```python
from build123d import *

# Parameters (mm, degrees)
ESQUISSE1_R             = 4
EXTRUSION1_DEPTH        = 5
ENL_V_MAT_EXTRU_1_DEPTH = 2
CONG_1_R                = 2.5


with BuildPart() as part:
    # Esquisse1 → Extrusion1 (new body)
    with BuildSketch(Plane.XY):
        with BuildLine():
            Line((-8, 0), (8, 0))
            ThreePointArc((8, 0), (10.121320344, 0.878679656), (11, 3))
            Line((11, 3), (11, 37))
            ThreePointArc((11, 37), (8, 40), (11, 43))
            Line((11, 43), (11, 78))
            ThreePointArc((11, 78), (10.121320344, 80.121320344), (8, 81))
            Line((8, 81), (-8, 81))
            ThreePointArc((-8, 81), (-10.121320344, 80.121320344), (-11, 78))
            Line((-11, 78), (-11, 3))
            ThreePointArc((-11, 3), (-10.121320344, 0.878679656), (-8, 0))
        make_face()
        with Locations((0, 9)):
            Circle(ESQUISSE1_R, mode=Mode.SUBTRACT)
        with Locations((0, 30)):
            Circle(ESQUISSE1_R, mode=Mode.SUBTRACT)
        with Locations((0, 50)):
            Circle(ESQUISSE1_R, mode=Mode.SUBTRACT)
        with Locations((0, 70)):
            Circle(ESQUISSE1_R, mode=Mode.SUBTRACT)
    extrude(amount=EXTRUSION1_DEPTH)

    # Esquisse2 → Enlèv. mat.-Extru.1 (cut)
    with BuildSketch(Plane.XY.offset(5)):
        with BuildLine():
            Line((4, 75.744562647), (4, 64.255437353))
            ThreePointArc((4, 64.255437353), (0, 63), (-4, 64.255437353))
            Line((-4, 64.255437353), (-4, 75.744562647))
            ThreePointArc((-4, 75.744562647), (0, 77), (4, 75.744562647))
        make_face()
    extrude(amount=-ENL_V_MAT_EXTRU_1_DEPTH, mode=Mode.SUBTRACT)

    # Congé1
    # the kernel refuses this fillet: 2.5 mm, written as the material it takes off along each edge
    with BuildSketch(Plane(origin=(11, -3.25, 0), x_dir=(0, 0, 1), z_dir=(0, 1, 0)), Plane(origin=(11, -3.25, 5), x_dir=(-1, 0, 0), z_dir=(0, 1, 0))) as cong_1_piece_1:
        with BuildLine():
            CenterArc((CONG_1_R, -CONG_1_R), CONG_1_R, 90, 90)
            Line((0, -CONG_1_R), (0, 0))
            Line((0, 0), (CONG_1_R, 0))
        make_face()
    extrude(amount=46.5, mode=Mode.SUBTRACT)
    with BuildSketch(Plane(origin=(-11, 84.25, 0), x_dir=(0, 0, 1), z_dir=(0, -1, 0))) as cong_1_piece_2:
        with BuildLine():
            CenterArc((CONG_1_R, -CONG_1_R), CONG_1_R, 90, 90)
            Line((0, -CONG_1_R), (0, 0))
            Line((0, 0), (CONG_1_R, 0))
        make_face()
    extrude(amount=87.5, mode=Mode.SUBTRACT)
    with BuildSketch(Plane(origin=(-11, 84.25, 5), x_dir=(0, 0, -1), z_dir=(0, -1, 0))) as cong_1_piece_3:
        with BuildLine():
            CenterArc((CONG_1_R, CONG_1_R), CONG_1_R, 180, 90)
            Line((0, CONG_1_R), (0, 0))
            Line((0, 0), (CONG_1_R, 0))
        make_face()
    extrude(amount=87.5, mode=Mode.SUBTRACT)
    with BuildSketch(Plane(origin=(11, 36.75, 0), x_dir=(0, 0, 1), z_dir=(0, 1, 0)), Plane(origin=(11, 36.75, 5), x_dir=(-1, 0, 0), z_dir=(0, 1, 0))) as cong_1_piece_4:
        with BuildLine():
            CenterArc((CONG_1_R, -CONG_1_R), CONG_1_R, 90, 90)
            Line((0, -CONG_1_R), (0, 0))
            Line((0, 0), (CONG_1_R, 0))
        make_face()
    extrude(amount=47.5, mode=Mode.SUBTRACT)


solid = part.part
```
Could you check a few things on this model? Use its own coordinates, in mm. A direction names the side the tool comes from. Round coordinates to 2 decimals unless told otherwise and drop trailing zeros. Write each loop counter-clockwise with the first axis right and the second up, starting at its lowest first coordinate (ties: lowest second). Pieces come first, ordered by that corner, then holes.
(1) Suppose I cut it at C-C on z = 0.75. Write out the boundary of the cut face in (x, y), and give its area (3 significant figures).
Findings below:
outline: (-10.29, 1.06) arc R3 ccw to (-8, 0) - (8, 0) arc R3 ccw to (10.29, 1.06) - (10.29, 37.09) arc R3 cw to (10.29, 42.91) - (10.29, 79.94) arc R3 ccw to (8, 81) - (-8, 81) arc R3 ccw to (-10.29, 79.94) - close; hole circle Ø8 at (0, 9); hole circle Ø8 at (0, 30); hole circle Ø8 at (0, 50); hole circle Ø8 at (0, 70)
area: 1,450 mm2
(2) Suppose I cut it at D-D on y = 14.5. Write out the boundary of the cut face in (x, z).
Findings below:
outline: (-8.5, 0) - (8.5, 0) arc R2.5 ccw to (8.5, 5) - (-8.5, 5) arc R2.5 ccw to start
(3) If I drill on probe 1 along Y at (x, z) = (0, 3.5); probe 2 along Y at (x, z) = (0, 2.6); probe 3 along Y at (x, z) = (-8.25, 4.6), over which ranges is the centre line in solid material (lowest first)?
Findings below:
probe 1: y = 0 to 5, 13 to 26, 34 to 46, 54 to 63, 77 to 81
probe 2: y = 0 to 5, 13 to 26, 34 to 46, 54 to 66, 74 to 81
probe 3: y = 0.01 to 80.99
(4) For pin 1 (10.5 mm diameter, centred on x = 0, y = 50, fed in from +Z); pin 2 (3.5 mm diameter, centred on x = 1, y = 73.5, fed in from +Z); pin 3 (1.6 mm diameter, centred on y = 72, z = 4.5, fed in from -X); pin 4 (2 mm diameter, centred on y = 72, z = 4.5, fed in from +X), each with a flat end and sliding along its axis, tell me the tip position at first contact or that it passes through.
Findings below:
pin 1: stops at z = 5
pin 2: stops at z = 3
pin 3: stops at x = -10.69
pin 4: stops at x = 10.79
(5) Thinking about a two-plate mould opening in Y: for faces 3 (the face through (9.748, 80.438, 2.465)), 4 (the face through (9.69, 0.52, 2.46)), 5 (the face through (-0.521, 33.966, 2.465)), which applies, +Y half, -Y half, draft (parallel to the pull), parting line (faces both ways), or undercut?
Findings below:
face 3: +Y half
face 4: -Y half
face 5: undercut
(6) Suppose I cut it at A-A on y = 50. Write out the boundary of the cut face in (x, z).
Findings below:
outline: (-8.5, 0) - (-4, 0) - (-4, 5) - (-8.5, 5) arc R2.5 ccw to start; (4, 0) - (8.5, 0) arc R2.5 ccw to (8.5, 5) - (4, 5) - close
(7) Which directions (+Z, -Z, +X, -X, +Y, -Y) give clear straight access to the entire face, cutting with the end or side of a thin tool? Please do faces 1 (the face through (0, 0, 2)), 2 (the face through (0, 65, 3)).
Findings below:
face 1: +Z, -Z, +X, -X, -Y
face 2: +Z
(8) Suppose I cut it at B-B on x = -2.75. Write out the boundary of the cut face in (y, z), and give its area (3 significant figures).
Findings below:
outline: (0, 0) - (6.1, 0) - (6.1, 5) - (0, 5) - close; (11.9, 0) - (27.1, 0) - (27.1, 5) - (11.9, 5) - close; (32.9, 0) - (47.1, 0) - (47.1, 5) - (32.9, 5) - close; (52.9, 0) - (67.1, 0) - (67.1, 3) - (63.56, 3) - (63.56, 5) - (52.9, 5) - close; (72.9, 0) - (81, 0) - (81, 5) - (76.44, 5) - (76.44, 3) - (72.9, 3) - close
area: 275 mm2
